Can you work these out from the model? Positions are in its coordinate system, mm. Face numbers are marked on the shaded views. A direction names the side the tool comes from. Give positions to 0.01 mm unless a question says otherwise; leave off trailing zeros. Order: outer loops, then holes, each group sorted by start corner. A loop starts at its lowest first (then second) coordinate and runs counter-clockwise, first axis right, second up. Notation, with made-up numbers: (-28, -34) - (16, -34) arc R34 cw to (16, 3) - close; hole circle Ø11 at (-12.5, 89.25). An arc over 180 degrees is marked (long way). Answer as a JSON object with one key per item and string values.
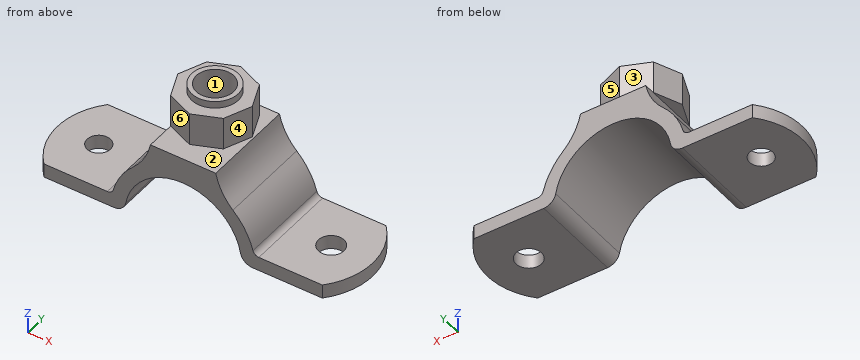
```python
from build123d import *

# Parameters (mm, degrees)
F1_DEPTH  = 10
F2_R      = 2.5
F2_R_2    = 2.7424095939
F3_DEPTH  = 25
F5_DEPTH  = 3
F7_DEPTH  = 3
F8_R      = 5
F9_DEPTH  = 2
F11_DEPTH = 7
F12_R     = 5
F12_R_2   = 4
F13_DEPTH = 1.5
F14_DEPTH = 11


with BuildPart() as f1:
    # F0 (on Front) → F1 (new body, symmetric)
    with BuildSketch(Plane.XZ):
        with BuildLine():
            ThreePointArc((-12.3133069376, 2.1523178808), (0, 12.5), (12.3133069376, 2.1523178808))
            ThreePointArc((12.3133069376, 2.1523178808), (13.2017484895, 0.6095259974), (14.8744747806, 0))
            Line((14.8744747806, 0), (29.85, 0))
            Line((29.85, 0), (29.85, 3))
            Line((29.85, 3), (16.2403817689, 3))
            ThreePointArc((16.2403817689, 3), (15.4474629596, 3.2698156661), (14.9836855606, 3.9672619048))
            ThreePointArc((14.9836855606, 3.9672619048), (13.3355324821, 7.9002261625), (10.6780077367, 11.2352192135))
            ThreePointArc((10.6780077367, 11.2352192135), (8.326658054, 14.3390474584), (7, 18))
            Line((7, 18), (-7, 18))
            ThreePointArc((-7, 18), (-8.326658054, 14.3390474584), (-10.6780077367, 11.2352192135))
            ThreePointArc((-10.6780077367, 11.2352192135), (-13.3355324821, 7.9002261625), (-14.9836855606, 3.9672619048))
            ThreePointArc((-14.9836855606, 3.9672619048), (-15.4474629596, 3.2698156661), (-16.2403817689, 3))
            Line((-16.2403817689, 3), (-29.85, 3))
            Line((-29.85, 3), (-29.85, 0))
            Line((-29.85, 0), (-14.8744747806, 0))
            ThreePointArc((-14.8744747806, 0), (-13.2017484895, 0.6095259974), (-12.3133069376, 2.1523178808))
        make_face()
    extrude(amount=F1_DEPTH, both=True)

    # F2 (on face) → F3 (cut)
    with BuildSketch(Plane.XY.offset(3)):
        with Locations((-24.92, 0)):
            Circle(F2_R)
        with Locations((24.92, 0)):
            Circle(F2_R_2)
    extrude(amount=-F3_DEPTH, mode=Mode.SUBTRACT)

    # F4 (on face) → F5 (join)
    with BuildSketch(Plane.XY.offset(3)):
        with BuildLine():
            Line((-29.85, -10), (-29.85, 10))
            ThreePointArc((-29.85, 10), (-33.7754930507, 0), (-29.85, -10))
        make_face()
    extrude(amount=-F5_DEPTH)

    # F6 (on face) → F7 (join)
    with BuildSketch(Plane.XY.offset(3)):
        with BuildLine():
            Line((29.85, 10), (29.85, -10))
            ThreePointArc((29.85, -10), (33.7754930507, 0), (29.85, 10))
        make_face()
    extrude(amount=-F7_DEPTH)

    # F8 (on face) → F9 (join)
    with BuildSketch(Plane.XY.offset(18)):
        Circle(F8_R)
    extrude(amount=F9_DEPTH)

    # F10 (on face) → F11 (join)
    with BuildSketch(Plane.XY.offset(20)):
        Polygon((5.6568542495, 5.6568542495), (0, 8), (-5.6568542495, 5.6568542495), (-8, 0), (-5.6568542495, -5.6568542495), (0, -8), (5.6568542495, -5.6568542495), (8, 0), align=None)
    extrude(amount=F11_DEPTH)

    # F12 (on face) → F13 (join)
    with BuildSketch(Plane.XY.offset(27)):
        Circle(F12_R)
        Circle(F12_R_2, mode=Mode.SUBTRACT)
    extrude(amount=F13_DEPTH)

    # F14 (cut): a face of the model
    f14_faces = [f1.faces().sort_by_distance(p)[0] for p in [
        (0, 0, 27),
    ]]
    extrude(f14_faces, amount=-F14_DEPTH, mode=Mode.SUBTRACT)


solid = f1.part
```
Q1. If we section it at C-C, the plane z = 5.5: Please give me the cut outline in (x, y), then the cut area to 3 significant figures.
Recorded:
{"outline": "(-14.49, -10) - (-11.22, -10) - (-11.22, 10) - (-14.49, 10) - close; (11.22, -10) - (14.49, -10) - (14.49, 10) - (11.22, 10) - close", "area": "131 mm^2"}
Q2. Which directions (+Z, -Z, +X, -X, +Y, -Y) give clear straight access to the entire face, cutting with the end or side of a thin tool? Please do the marked faces 4, 5 and 6.
Recorded:
{"face 4": "+Z, +X, -Y", "face 5": "+Z, +X, +Y", "face 6": "+Z, -X, -Y"}
Q3. I need wall thicknesses on L1, parallel to Y at x = 24.92, z = 1.75; L2, parallel to Y at x = -24.92, z = 1.05; L3, parallel to Z at x = -17.5, y = 5.25. Which ranges of each line are inside material? Lowest first, please.
Recorded:
{"L1": "y = -10 to -2.74, 2.74 to 10", "L2": "y = -10 to -2.5, 2.5 to 10", "L3": "z = 0 to 3"}
Q4. If we section it at D-D, the plane y = 6.5: Please give me the cut outline in (x, z).
Recorded:
{"outline": "(-32.26, 0) - (-14.87, 0) arc R2.6 ccw to (-12.31, 2.15) arc R12.5 cw to (12.31, 2.15) arc R2.6 ccw to (14.87, 0) - (32.26, 0) - (32.26, 3) - (16.24, 3) arc R1.3 cw to (14.98, 3.97) arc R15.5 ccw to (10.68, 11.24) arc R13 cw to (7, 18) - (-7, 18) arc R13 cw to (-10.68, 11.24) arc R15.5 ccw to (-14.98, 3.97) arc R1.3 cw to (-16.24, 3) - (-32.26, 3) - close; (-3.62, 20) - (3.62, 20) - (3.62, 27) - (-3.62, 27) - close"}
Q5. If we section it at A-A, the plane x = -24.92: Please give me the cut outline in (y, z).
Recorded:
{"outline": "(-10, 0) - (-2.5, 0) - (-2.5, 3) - (-10, 3) - close; (2.5, 0) - (10, 0) - (10, 3) - (2.5, 3) - close"}
Q6. If we section it at B-B, the plane z = 24: Please give me the cut outline in (x, y).
Recorded:
{"outline": "(-8, 0) - (-5.66, -5.66) - (0, -8) - (5.66, -5.66) - (8, 0) - (5.66, 5.66) - (0, 8) - (-5.66, 5.66) - close; hole circle Ø8 at (0, 0)"}
Q7. We'd pull the mould along Y, two halves only. Please class the marked faces 1, 2 and 3: released by +Y, released by -Y, zero draft, split by the parting line, or undercut.
Recorded:
{"face 1": "undercut", "face 2": "zero draft", "face 3": "released by +Y"}
Q8. I'm going to push flat-ended pins straight in: pin 1 Ø2 at (y, z) = (-7.5, 17.5) entering from +X; pin 2 Ø1 at (y, z) = (4, 16.5) entering from +X; pin 3 Ø9 at (x, y) = (-24.5, 3.5) entering from +Z. Where does each tip first touch, or does it pass through?
Recorded:
{"pin 1": "stops at x = 7.39", "pin 2": "stops at x = 7.57", "pin 3": "stops at z = 3"}
